from build123d import *

# Parameters (mm, degrees)
ESQUISSE1_W                  = 9
ESQUISSE1_H                  = 3.146636507
ESQUISSE2_W                  = 7.05
ESQUISSE2_H                  = 3.5
R_P_TITION_CIRCULAIRE1_COUNT = 15


with BuildPart() as part:
    # Esquisse1 → Base-Révolution (revolve)
    with BuildSketch(Plane.XY, mode=Mode.PRIVATE) as base_r_volution_sk:
        with Locations((-1.139387669, 23.073318253)):
            Rectangle(ESQUISSE1_W, ESQUISSE1_H)
    revolve(base_r_volution_sk.sketch.rotate(Axis((-8.771095324, 0, 0), (1, 0, 0)), 90), axis=Axis((-8.771095324, 0, 0), (1, 0, 0)))

    # Esquisse2 → Enlèvement de matière-Révolution1 (revolve, cut)
    with BuildSketch(Plane.XY):
        with Locations((-0.951181968, 25.25)):
            Rectangle(ESQUISSE2_W, ESQUISSE2_H)
    enl_vement_de_mati_re_r_volution1 = revolve(axis=Axis((-7.697366985, 23.5, 0), (1, 0, 0)), mode=Mode.SUBTRACT)

    # Répétition circulaire1: Enlèvement de matière-Révolution1 ×15 about axis
    r_p_tition_circulaire1_axis = Axis((0, 0, 0), (1, 0, 0))
    for i in range(1, R_P_TITION_CIRCULAIRE1_COUNT):
        add(enl_vement_de_mati_re_r_volution1.rotate(r_p_tition_circulaire1_axis, i * 360 / R_P_TITION_CIRCULAIRE1_COUNT), mode=Mode.SUBTRACT)


solid = part.part
For this review, take the finished solid that the model builds, in its own axes (mm). A direction names the side the tool comes from. Give positions to 0.01 mm unless a question says otherwise; leave off trailing zeros. Loops run counter-clockwise (first coordinate to the right, second up) from the corner with the lowest first, then second, coordinate; pieces in that order, holes last. Notation, with made-up numbers: M 83.5,-20.5 L 121.5,-20.5 A23 cw 121.5,-2.5 Z; hole C 13.25,84 d6. An arc over 180 degrees is marked long. Put each result on its own line as item: value. Start each with the question number.
(1) Add section D-D, the plane x = 1. Give the number of separate pieces and of enclosed holes in the cut face, then the cut area to 3 significant figures.
(2) The part is to be moulded in two halves that separate along X. For faces 1 (the cylindrical face through (-0.9, -5.8, 22.33)), 2 (the flat face through (-5.639, -22, -2)), say which applies: +X half, -X half, draft (parallel to the pull), parting line (faces both ways), or undercut.
(3) For pin 1 (5 mm diameter, centred on x = -1.5, z = 10, fed in from +Y); pin 2 (5 mm diameter, centred on x = -4.5, y = 4.5, fed in from -Z); pin 3 (3 mm diameter, centred on x = -3.5, z = 8.5, fed in from -Y), all flat-tipped, find the tip position at first contact; note any pin that passes through.
(4) Add section C-C, the plane y = 19.5. Write out the cut boundary in (x, z), then the cut area to 3 significant figures.
(5) Add section A-A, the plane z = 0. Write out the cut boundary in (x, y).
(6) Wall thickness on L1, parallel to Y at x = -3.5, z = -22; L2, parallel to Y at x = -1.5, z = 0; L3, parallel to X at y = -22, z = -2.5: over which ranges is each line inside the solid? List them lowest first.
(7) Add section B-B, the plane y = -3. Write out the cut boundary in (x, z), then the cut area to 3 significant figures.
(8) Machinability: for faces 3 (the cylindrical face through (-0.902, -20.476, 10.634)), 4 (the cylindrical face through (-0.9, -8.42, 21.43)), 5 (the flat face through (2.574, -19, -14)), which of the approach directions +Z, -Z, +X, -X, +Y, -Y give a long, thin tool a straight path to every point of the face, cutting with its end or side? Answer none if there is none.
Result:
1. separate pieces: 15
1. enclosed holes: 0
1. area: 142 mm^2
2. face 1: undercut
2. face 2: -X half
3. pin 1: stops at y = 19.57
3. pin 2: stops at z = -24.57
3. pin 3: stops at y = -23.52
4. outline: M -5.64,-15.07 L 3.36,-15.07 L 3.36,-9.06 L 2.57,-9.06 L 2.57,-12.45 L -4.48,-12.45 L -4.48,-9.06 L -5.64,-9.06 Z; M -5.64,9.06 L -4.48,9.06 L -4.48,12.45 L 2.57,12.45 L 2.57,9.06 L 3.36,9.06 L 3.36,15.07 L -5.64,15.07 Z
4. area: 60.4 mm^2
5. outline: M -5.64,-24.65 L 3.36,-24.65 L 3.36,-21.5 L -5.64,-21.5 Z; M -5.64,21.5 L -4.48,21.5 L -4.48,24.65 L -5.64,24.65 Z; M 2.57,21.5 L 3.36,21.5 L 3.36,24.65 L 2.57,24.65 Z
6. L1: y = -8.66 to -5.68, 0.76 to 3.78, 10.74 to 11.11
6. L2: y = -24.65 to -21.5
6. L3: x = -5.64 to -4.48, 2.57 to 3.36
7. outline: M -5.64,-24.46 L -4.48,-24.46 L -4.48,-21.29 L -5.64,-21.29 Z; M -5.64,21.29 L -4.48,21.29 L -4.48,24.46 L -5.64,24.46 Z; M 2.57,-24.46 L 3.36,-24.46 L 3.36,-21.29 L 2.57,-21.29 Z; M 2.57,21.29 L 3.36,21.29 L 3.36,24.46 L 2.57,24.46 Z
7. area: 12.4 mm^2
8. face 3: +Z
8. face 4: -Y
8. face 5: none
